Check sheet for the modelled part. Datum: model origin and axes. Units: mm. Give positions to 0.01 mm unless a question says otherwise; leave off trailing zeros. Order: outer loops, then holes, each group sorted by start corner. A loop starts at its lowest first (then second) coordinate and runs counter-clockwise, first axis right, second up.
```python
from build123d import *

# Parameters (mm, degrees)
F1_DEPTH = 25


with BuildPart() as f1:
    # F0 (on Top) → F1 (new body)
    with BuildSketch(Plane.XY):
        with BuildLine():
            Line((-300, 0), (300, 0))
            ThreePointArc((300, 0), (0, 300), (-300, 0))
        make_face()
        with BuildLine():
            Line((-11.572157, 30), (-257.588138, 30))
            ThreePointArc((-257.588138, 30), (-231.676934, 116.522303), (-177.663751, 188.910668))
            Line((-177.663751, 188.910668), (-110.826445, 124.963055))
            Line((-110.826445, 124.963055), (-11.572157, 30))
        make_face(mode=Mode.SUBTRACT)
        with BuildLine():
            ThreePointArc((169.856684, 195.960087), (229.266126, 121.196915), (257.588138, 30))
            Line((257.588138, 30), (11.071837, 30))
            Line((11.071837, 30), (96.545549, 119.336136))
            Line((96.545549, 119.336136), (169.856684, 195.960087))
        make_face(mode=Mode.SUBTRACT)
        with BuildLine():
            Line((-7, 46.385215), (-100.456727, 135.801364))
            Line((-100.456727, 135.801364), (-166.405643, 198.898996))
            ThreePointArc((-166.405643, 198.898996), (-91.801305, 242.536944), (-7, 259.234737))
            Line((-7, 259.234737), (-7, 211.881727))
            Line((-7, 211.881727), (-7, 46.385215))
        make_face(mode=Mode.SUBTRACT)
        with BuildLine():
            Line((158.447307, 205.295153), (8, 48.049365))
            Line((8, 48.049365), (8, 211.881727))
            Line((8, 211.881727), (8, 259.205804))
            ThreePointArc((8, 259.205804), (87.48009, 244.128824), (158.447307, 205.295153))
        make_face(mode=Mode.SUBTRACT)
    extrude(amount=F1_DEPTH)


solid = f1.part
```
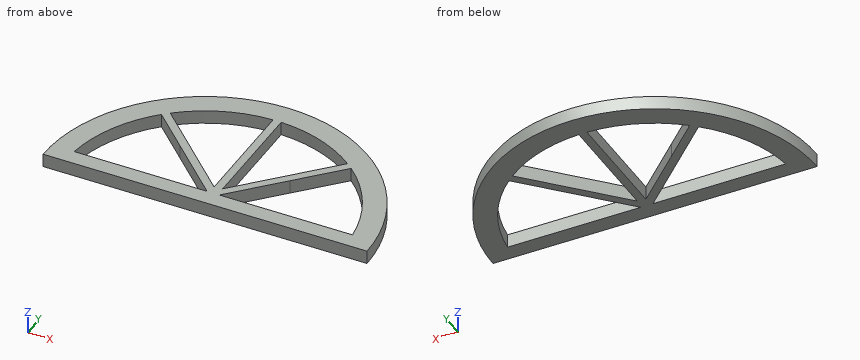
(1) Sectioned sample at B-B (y = 244). Enter the section's corners in (x, z).
(2) Thickness scan on L1, parallel to Y at x = 129, z = 4.25; L2, parallel to Y at x = -154.5, z = 15; L3, parallel to X at y = 41, z = 14.75. Record the ranges inside material, lowest first.
(3) Go/stop test with flat-tipped pins: P1, Ø1.5, axis at y = 226.5, z = 18, coming from the -X side; P2, Ø12.5, axis at y = 160, z = 9.5, coming from the +X side; P3, Ø12.5, axis at y = 114, z = 16.5, coming from the -X side. Record where each tip stops, or that it passes through.
(4) Sectioned sample at D-D (y = 60). Enter the section's corners in (x, z), plus the area to 3 significant figures.
(5) Sectioned sample at C-C (x = 53.5). Enter the section's corners in (y, z).
(6) Sectioned sample at A-A (z = 16.75). Enter the section's corners in (x, y).
Values follow:
1. outline: (-174.54, 0) - (-87.84, 0) - (-87.84, 25) - (-174.54, 25) - close; (-7, 0) - (8, 0) - (8, 25) - (-7, 25) - close; (87.84, 0) - (174.54, 0) - (174.54, 25) - (87.84, 25) - close
2. L1: y = 0 to 30, 153.26 to 174.52, 224.97 to 270.85
2. L2: y = 0 to 30, 166.75 to 187.51, 208.28 to 257.16
2. L3: x = -297.19 to -256.07, -23.07 to 21.6, 256.07 to 297.19
3. P1: stops at x = -197.58
3. P2: stops at x = 257.61
3. P3: stops at x = -279.98
4. outline: (-293.94, 0) - (-252.29, 0) - (-252.29, 25) - (-293.94, 25) - close; (-42.93, 0) - (-21.23, 0) - (-21.23, 25) - (-42.93, 25) - close; (-7, 0) - (8, 0) - (8, 25) - (-7, 25) - close; (19.43, 0) - (39.77, 0) - (39.77, 25) - (19.43, 25) - close; (252.29, 0) - (293.94, 0) - (293.94, 25) - (252.29, 25) - close
4. area: 3,510 mm2
5. outline: (0, 0) - (30, 0) - (30, 25) - (0, 25) - close; (74.35, 0) - (95.61, 0) - (95.61, 25) - (74.35, 25) - close; (253.75, 0) - (295.19, 0) - (295.19, 25) - (253.75, 25) - close
6. outline: (-300, 0) - (300, 0) arc R300 ccw to start; hole (-257.59, 30) - (-11.57, 30) - (-177.66, 188.91) arc R259.33 ccw to start; hole (-166.41, 198.9) - (-7, 46.39) - (-7, 259.23) arc R259.33 ccw to start; hole (8, 48.05) - (158.45, 205.3) arc R259.33 ccw to (8, 259.21) - close; hole (11.07, 30) - (257.59, 30) arc R259.33 ccw to (169.86, 195.96) - close
